```python
from build123d import *

# Parameters (mm, degrees)
F1_DEPTH = 5
F2_W     = 50
F2_H     = 10
F3_DEPTH = 20
F4_W     = 50
F4_H     = 95
F5_DEPTH = 5


with BuildPart() as f1:
    # F0 (on Top) → F1 (new body)
    with BuildSketch(Plane.XY):
        with BuildLine():
            Line((-23, -100), (23, -100))
            ThreePointArc((23, -100), (24.414214, -99.414214), (25, -98))
            Line((25, -98), (25, 98))
            ThreePointArc((25, 98), (24.414214, 99.414214), (23, 100))
            Line((23, 100), (-23, 100))
            ThreePointArc((-23, 100), (-24.414214, 99.414214), (-25, 98))
            Line((-25, 98), (-25, 60))
            ThreePointArc((-25, 60), (-24.414214, 58.585786), (-23, 58))
            Line((-23, 58), (-4.25, 58))
            ThreePointArc((-4.25, 58), (-3.542893, 58.292893), (-3.25, 59))
            Line((-3.25, 59), (-3.25, 65))
            ThreePointArc((-3.25, 65), (0, 68.25), (3.25, 65))
            Line((3.25, 65), (3.25, 54.75))
            ThreePointArc((3.25, 54.75), (2.298097, 52.451903), (0, 51.5))
            Line((0, 51.5), (-23, 51.5))
            ThreePointArc((-23, 51.5), (-24.414214, 50.914214), (-25, 49.5))
            Line((-25, 49.5), (-25, -70))
            ThreePointArc((-25, -70), (-24.414214, -71.414214), (-23, -72))
            Line((-23, -72), (-4.25, -72))
            ThreePointArc((-4.25, -72), (-3.542893, -71.707107), (-3.25, -71))
            Line((-3.25, -71), (-3.25, -65))
            ThreePointArc((-3.25, -65), (0, -61.75), (3.25, -65))
            Line((3.25, -65), (3.25, -75.25))
            ThreePointArc((3.25, -75.25), (2.298097, -77.548097), (0, -78.5))
            Line((0, -78.5), (-23, -78.5))
            ThreePointArc((-23, -78.5), (-24.414214, -79.085786), (-25, -80.5))
            Line((-25, -80.5), (-25, -98))
            ThreePointArc((-25, -98), (-24.414214, -99.414214), (-23, -100))
        make_face()
    extrude(amount=F1_DEPTH)

    # F2 (on face) → F3 (join)
    with BuildSketch(Plane(origin=(0, 0, 0), x_dir=(1, 0, 0), z_dir=(0, 0, -1))):
        with BuildLine():
            Line((10, 25), (-10, 25))
            ThreePointArc((-10, 25), (-17.5, 17.5), (-10, 10))
            Line((-10, 10), (10, 10))
            ThreePointArc((10, 10), (17.5, 17.5), (10, 25))
        make_face()
        with BuildLine():
            Line((10, -5), (-10, -5))
            ThreePointArc((-10, -5), (-17.5, -12.5), (-10, -20))
            Line((-10, -20), (10, -20))
            ThreePointArc((10, -20), (17.5, -12.5), (10, -5))
        make_face()
        with Locations((0, 45)):
            Rectangle(F2_W, F2_H)
        with Locations((0, -40)):
            Rectangle(F2_W, F2_H)
    extrude(amount=F3_DEPTH)

    # F4 (on face) → F5 (join)
    with BuildSketch(Plane(origin=(0, 0, -20), x_dir=(1, 0, 0), z_dir=(0, 0, -1))):
        with Locations((0, 2.5)):
            Rectangle(F4_W, F4_H)
    extrude(amount=F5_DEPTH)


solid = f1.part
```
Build history of the part. All positions in model axes, mm. A direction names the side the tool comes from. Give positions to 0.01 mm unless a question says otherwise; leave off trailing zeros. Loops run counter-clockwise (first coordinate to the right, second up) from the corner with the lowest first, then second, coordinate; pieces in that order, holes last. Notation, with made-up numbers: (66, -4) - (94, -4) arc R17 ccw to (94, 14) - close; hole circle Ø11 at (9.25, -0.5). An arc over 180 degrees is marked (long way). Use a Markdown table: item, result.
(1) Wall check: line 1 along Y through (x, z) = (-9, -2); line 2 along Y through (x, z) = (-15, 3.75); line 3 along Z through (x, y) = (22.5, 33). Give the ranges that are in metal, low to high.
Taken from the geometry:
| item | result |
|---|---|
| line 1 | -50 to -40, -25 to -10, 5 to 20, 35 to 45 |
| line 2 | -100 to -78.5, -72 to 51.5, 58 to 100 |
| line 3 | -25 to -20, 0 to 5 |
(2) Band-saw the part on C-C (x = 7). Give the cut face in (y, z), and give its area (4 significant figures).
Taken from the geometry:
| item | result |
|---|---|
| outline | (-100, 0) - (-50, 0) - (-50, -25) - (45, -25) - (45, 0) - (100, 0) - (100, 5) - (-100, 5) - close; hole (-40, -20) - (-25, -20) - (-25, 0) - (-40, 0) - close; hole (-10, -20) - (5, -20) - (5, 0) - (-10, 0) - close; hole (20, -20) - (35, -20) - (35, 0) - (20, 0) - close |
| area | 2,475 mm2 |
(3) Band-saw the part on D-D (y = 12.5). Give the cut face in (x, z).
Taken from the geometry:
| item | result |
|---|---|
| outline | (-25, -25) - (25, -25) - (25, -20) - (17.5, -20) - (17.5, 0) - (25, 0) - (25, 5) - (-25, 5) - (-25, 0) - (-17.5, 0) - (-17.5, -20) - (-25, -20) - close |
(4) Pull direction Z, two halves, no side cores. Call faces 1 (the face through (-11, -78.5, 2)), 2 (the face through (0, -3, -20)), 3 (the face through (5, -75, 0)): +Z half, -Z half, draft (parallel to the pull), parting line (faces both ways), or undercut.
Taken from the geometry:
| item | result |
|---|---|
| face 1 | draft |
| face 2 | undercut |
| face 3 | -Z half |
(5) Which spindle directions (+Z, -Z, +X, -X, +Y, -Y) get a long thin tool onto all of the face, cutting with end or side? Do faces 4 (the face through (-14, 58, 2)), 5 (the face through (-3.25, 62, 2)), 6 (the face through (0, 5, -10)), 7 (the face through (0, -50, -12)). Say none if no direction does.
Taken from the geometry:
| item | result |
|---|---|
| face 4 | +Z, -Z, -X |
| face 5 | +Z, -Z |
| face 6 | +X, -X |
| face 7 | -Z, +X, -X, -Y |
(6) Drop flat-ended pins along their axis: pin 1 Ø25 at (x, y) = (-5, -68) entering from -Z; pin 2 Ø6 at (x, z) = (-8, -12.5) entering from +Y; pin 3 Ø6 at (y, z) = (-54, -8) entering from +X; pin 4 Ø10 at (x, z) = (5, -6.5) entering from -Y. Give the stop position or say it passes through.
Taken from the geometry:
| item | result |
|---|---|
| pin 1 | z = 0 |
| pin 2 | y = 45 |
| pin 3 | through |
| pin 4 | y = -50 |
(7) Band-saw the part on A-A (z = -8). Give the cut face in (x, y), and give its area (3 significant figures).
Taken from the geometry:
| item | result |
|---|---|
| outline | (-25, -50) - (25, -50) - (25, -40) - (-25, -40) - close; (-25, 35) - (25, 35) - (25, 45) - (-25, 45) - close; (-10, -25) - (10, -25) arc R7.5 ccw to (10, -10) - (-10, -10) arc R7.5 ccw to start; (-10, 5) - (10, 5) arc R7.5 ccw to (10, 20) - (-10, 20) arc R7.5 ccw to start |
| area | 1,950 mm2 |
(8) Band-saw the part on B-B (y = -31). Give the cut face in (x, z).
Taken from the geometry:
| item | result |
|---|---|
| outline | (-25, -25) - (25, -25) - (25, -20) - (-25, -20) - close; (-25, 0) - (25, 0) - (25, 5) - (-25, 5) - close |
